from build123d import *

# Parameters (mm, degrees)
F0_W     = 75
F0_H     = 25
F1_DEPTH = 15
F2_SIZE  = 10
F3_SIZE  = 10
F4_R     = 5
F5_R     = 5
F6_R     = 4.99999


# Not quite as in the source:
# - a fillet or chamfer is up to 0.001 mm smaller than in the source, because OpenCascade refuses the exact size


with BuildPart() as f1:
    # F0 (on Right) → F1 (new body)
    with BuildSketch(Plane.YZ):
        Rectangle(F0_W, F0_H)
    extrude(amount=F1_DEPTH)

    # F2
    f2_edges = [f1.edges().sort_by_distance(p)[0] for p in [
        (7.5, -37.5, 12.5),
    ]]
    chamfer(f2_edges, length=F2_SIZE)

    # F3
    f3_edges = [f1.edges().sort_by_distance(p)[0] for p in [
        (7.5, -37.5, -12.5),
    ]]
    chamfer(f3_edges, length=F3_SIZE)

    # F4
    f4_edges = [f1.edges().sort_by_distance(p)[0] for p in [
        (15, 5, 12.5),
        (0, 5, 12.5),
        (15, 5, -12.5),
        (0, 5, -12.5),
    ]]
    fillet(f4_edges, radius=F4_R)

    # F5
    f5_edges = [f1.edges().sort_by_distance(p)[0] for p in [
        (7.5, 37.5, -12.5),
        (1.464466, 37.5, -11.035534),
        (13.535534, 37.5, -11.035534),
        (0, 37.5, 0),
        (15, 37.5, 0),
        (1.464466, 37.5, 11.035534),
        (13.535534, 37.5, 11.035534),
        (7.5, 37.5, 12.5),
    ]]
    fillet(f5_edges, radius=F5_R)

    # F6 (radius 5 in the source; OpenCascade refuses exactly that, so slightly less here)
    f6_edges = [f1.edges().sort_by_distance(p)[0] for p in [
        (0, -37.5, 0),
        (7.5, -37.5, -2.5),
        (7.5, -37.5, 2.5),
        (15, -37.5, 0),
    ]]
    fillet(f6_edges, radius=F6_R)


solid = f1.part
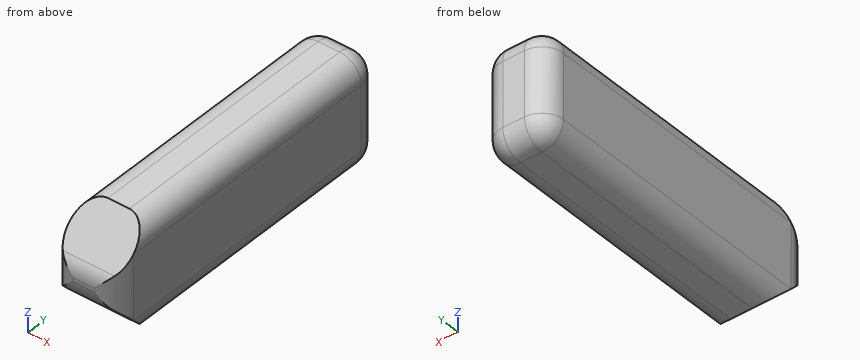
Build history of the part. All positions in model axes, mm. Round coordinates to 2 decimals unless told otherwise and drop trailing zeros. Loops run counter-clockwise (first coordinate to the right, second up) from the corner with the lowest first, then second, coordinate; pieces in that order, holes last. Notation, with made-up numbers: (48.25, -33) -> (57.25, -33) arc R27 ccw to (57.25, 0) -> close; hole circle Ø5 at (77, -11). An arc over 180 degrees is marked (long way). Use CSV: the item, a comma, the result in double quotes. Start each with the question number.
Q1. Flat gauge pins, fed straight in: pin 1 Ø3 at (x, z) = (13.5, -3) entering from +Y; pin 2 Ø1.5 at (x, z) = (8.5, 9.5) entering from -Y; pin 3 Ø5 at (x, y) = (13, 0) entering from +Z. Where does each tip first touch, or does it go through?
Q2. Drill centre lines: L1, parallel to Y at x = 10, z = -7.5; L2, parallel to X at y = 20, z = -7.75; L3, parallel to X at y = 9.5, z = 9.75. Where is each one in solid material? Low to high.
Q3. Saw through at B-B on x = 6.75. Give the cut face in (y, z), and give its area (3 significant figures).
Q4. Saw through at C-C on z = -4.75. Give the cut face in (x, y).
Q5. Saw through at A-A on y = -29.5. Give the cut face in (x, z).
Q6. Saw through at D-D on x = 12. Give the cut face in (y, z), and give its area (3 significant figures).
Solutions:
1,pin 1,"stops at y = 37.08"
1,pin 2,"stops at y = -31.25"
1,pin 3,"stops at z = 12.47"
2,L1,"y = -32.5 to 37.5"
2,L2,"x = 0.01 to 14.99"
2,L3,"x = 0.53 to 14.47"
3,outline,"(-37.5, -0.43) arc R5 ccw to (-36.04, -3.96) -> (-27.5, -12.5) -> (32.5, -12.5) arc R5 ccw to (37.5, -7.5) -> (37.5, 7.5) arc R5 ccw to (32.5, 12.5) -> (-27.5, 12.5) -> (-36.04, 3.96) arc R5 ccw to (-37.5, 0.43) -> close"
3,area,"1,760 mm^2"
4,outline,"(0, -32.5) arc R5 ccw to (0.82, -35.25) -> (14.18, -35.25) arc R5 ccw to (15, -32.5) -> (15, 32.5) arc R5 ccw to (10, 37.5) -> (5, 37.5) arc R5 ccw to (0, 32.5) -> close"
5,outline,"(0, -7.5) arc R5 ccw to (1, -10.5) -> (14, -10.5) arc R5 ccw to (15, -7.5) -> (15, 7.5) arc R5 ccw to (14, 10.5) -> (1, 10.5) arc R5 ccw to (0, 7.5) -> close"
6,outline,"(-37.08, -2.43) arc R5 ccw to (-36.04, -3.96) -> (-27.92, -12.08) -> (32.5, -12.08) arc R4.58 ccw to (37.08, -7.5) -> (37.08, 7.5) arc R4.58 ccw to (32.5, 12.08) -> (-27.92, 12.08) -> (-36.04, 3.96) arc R5 ccw to (-37.08, 2.43) -> close"
6,area,"1,700 mm^2"
